Autodesk Inventor part; units mm, degrees
ref_plane "YZ Plane" through (0, 0, 0) normal (1, 0, 0) x (0, 1, 0)
ref_plane "XZ Plane" through (0, 0, 0) normal (0, 1, 0) x (-1, 0, 0)
ref_plane "XY Plane" through (0, 0, 0) normal (0, 0, 1) x (1, 0, 0)
sketch "Sketch1" plane through (0, 0, 0) normal (0, 0, 1) x (1, 0, 0)
  arc A0 (-0.8035, 3.4065) -> (-0.6457, -3.4399) centre (0, 0) ccw
  arc A1 (66.6791, -16.0777) -> (65.8677, 19.1325) centre (70, 1.6133) ccw
  line L0 (-0.8035, 3.4065) -> (65.8677, 19.1325)
  line L1 (66.6791, -16.0777) -> (-0.6457, -3.4399)
  line L2 (0, 0) -> (70, 1.6133) construction
  line L3 (65.7529, 19.6192) -> (-0.9183, 3.8932)
  arc A2 (-0.9183, 3.8932) -> (-0.738, -3.9313) centre (0, 0) ccw
  line L4 (-0.738, -3.9313) -> (66.5869, -16.5692)
  arc A3 (66.5869, -16.5692) -> (65.7529, 19.6192) centre (70, 1.6133) ccw
  circle A4 centre (0, 0) radius 3.5 construction
  circle A5 centre (70, 1.6133) radius 18 construction
  dimension "d0" = 0.5
extrude "Extrusion1" add sketch "Sketch1" along normal blind 3.4
properties part number "Rubberband"
Model file for the job. Use its own axes, mm. A direction names the side the tool comes from. Coordinates: 2 decimals unless noted, no trailing zeros. Write each loop counter-clockwise with the first axis right and the second up, starting at its lowest first coordinate (ties: lowest second). Pieces come first, ordered by that corner, then holes. Notation, with made-up numbers: (-16.75, 10.25) - (24.25, 10.25) arc R30 cw to (24.25, 43.25) - close; hole circle Ø1 at (80.25, -35). An arc over 180 degrees is marked (long way). One line per item, written item: value. Start each with the question number.
1. Probe line 1 (Y direction, x = 70, z = 0.7); line 2 (Y direction, x = 27, z = 0.4); line 3 (X direction, y = -2, z = 0.5). List the from-to ranges inside material, lowest first. Write a range as from..to.
2. Slice it at A-A (y = 0). Write the cut outline in (x, z), plus the area to 3 significant figures.
3. Slice it at C-C (x = 16). Write the cut outline in (y, z), plus the area to 3 significant figures.
4. Tool access for faces 5 (the cylindrical face through (-3.5, -0.1, 1.7)), 6 (the flat face through (31.8, 11.3, 0)): list every direction of +Z, -Z, +X, -X, +Y, -Y with a clear straight run to the whole face (end or side of a thin tool).
5. Slice it at B-B (z = 1.45). Write the cut outline in (x, y), plus the area to 3 significant figures.
6. Mould opens along X. For faces 1 (the flat face through (31.8, 11.3, 3.4)), 2 (the flat face through (32.07, 11.16, 1.68)), 3 (the flat face through (32.884, 11.866, 1.676)), 4 (the flat face through (33.488, -9.847, 1.676)) say: released by +X, released by -X, zero draft, split by the parting line, or undercut.
Answers below:
1. line 1: y = -16.89..-16.39, 19.61..20.11
1. line 2: y = -9.14..-8.63, 9.96..10.48
1. line 3: x = -3.46..-2.87, 87.63..88.14
2. outline: (-4, 0) - (-3.5, 0) - (-3.5, 3.4) - (-4, 3.4) - close; (87.93, 0) - (88.43, 0) - (88.43, 3.4) - (87.93, 3.4) - close
2. area: 3.41 mm^2
3. outline: (-7.07, 0) - (-6.56, 0) - (-6.56, 3.4) - (-7.07, 3.4) - close; (7.37, 0) - (7.88, 0) - (7.88, 3.4) - (7.37, 3.4) - close
3. area: 3.48 mm^2
4. face 5: +Z, -Z
4. face 6: -Z, +X, -X, +Y, -Y
5. outline: (-0.92, 3.89) arc R4 ccw to (-0.74, -3.93) - (66.59, -16.57) arc R18.5 ccw (long way) to (65.75, 19.62) - close; hole (-0.8, 3.41) arc R3.5 ccw to (-0.65, -3.44) - (66.68, -16.08) arc R18 ccw (long way) to (65.87, 19.13) - close
5. area: 106 mm^2
6. face 1: zero draft
6. face 2: undercut
6. face 3: released by -X
6. face 4: undercut
